Read the model definition and answer for the solid it produces. Units are mm, in the model's axes. Face numbers are marked on the shaded views. A direction names the side the tool comes from. Coordinates: 2 decimals unless noted, no trailing zeros. Write each loop counter-clockwise with the first axis right and the second up, starting at its lowest first coordinate (ties: lowest second). Pieces come first, ordered by that corner, then holes. Notation, with made-up numbers: (54, 1.5) -> (85, 1.5) arc R25 cw to (85, 30.5) -> close; hole circle Ø11 at (89, 28.5). An arc over 180 degrees is marked (long way). Answer as a JSON object with one key per item and string values. Group by question number.
(1) Which of the six approach directions +Z, -Z, +X, -X, +Y, -Y give full straight-line access (tool end or side, diameter ignored) to the marked faces 1, 2, 3, 4 and 5?
(2) Flat-ended cylindrical pins translate along their axes: P1, Ø16, axis at y = -88.5, z = 18.5, coming from the +X side; P2, Ø3, axis at y = 41, z = 138.5, coming from the -X side; P3, Ø16, axis at x = 71, z = 15, coming from the -Y side. Find the tip coordinate at first contact, or state that the pin passes through.
(3) For a pull along X with two mould halves and no side action, classify the marked faces 6, 7, 8 and 9 as +X half, -X half, draft (parallel to the pull), parting line (faces both ways), or undercut.
(4) Find section D-D (x = -63.5). Give the vertices of the cut face in (y, z), then the cut area to 3 significant figures.
(5) Find section B-B (x = 75). Give the vertices of the cut face in (y, z).
(6) Find section C-C (z = 61). Give the vertices of the cut face in (x, y).
(7) Straight lines are drawn through the part: L1, parallel to Y at x = 75, z = 11; L2, parallel to X at y = -82, z = 32; L3, parallel to Z at x = 76, y = 56. For each, find the intervals that lie inside material, in ascending order.
(8) Find section A-A (y = -82.5). Give the vertices of the cut face in (x, z), then the cut area to 3 significant figures.
from build123d import *

# Parameters (mm, degrees)
F0_W            = 210
F0_H            = 225
F1_DEPTH        = 25
F3_DEPTH        = 95
F4_R            = 37.5
F5_DEPTH        = 10
F5_DEPTH_BACK   = 127
F6_R            = 40
F7_DEPTH        = 10
F7_DEPTH_BACK   = 127
F8_W            = 60
F8_H            = 60
F9_DEPTH        = 10
F10_R           = 10
F12_DEPTH       = 20
F14_D           = 15
F14_CBORE_D     = 30
F14_CBORE_DEPTH = 10
F15_R           = 10
F16_R           = 19.5
F17_DEPTH       = 235.001
F18_R           = 19.5
F19_DEPTH       = 220.001
F20_SIZE        = 2
F21_R           = 10


with BuildPart() as f1:
    # F0 (on Top) → F1 (new body)
    with BuildSketch(Plane.XY):
        Rectangle(F0_W, F0_H)
    extrude(amount=F1_DEPTH)

    # F2 (on face) → F3 (join)
    with BuildSketch(Plane.XY.offset(25)):
        with BuildLine():
            Line((-71, -32.5), (-71, -112.5))
            Line((-71, -112.5), (-56, -112.5))
            Line((-56, -112.5), (-56, -46.481817))
            ThreePointArc((-56, -46.481817), (7.488853, -14.988853), (38.981817, 48.5))
            Line((38.981817, 48.5), (105, 48.5))
            Line((105, 48.5), (105, 63.5))
            Line((105, 63.5), (25, 63.5))
            ThreePointArc((25, 63.5), (-3.117749, -4.382251), (-71, -32.5))
        make_face()
    extrude(amount=F3_DEPTH)

    # F4 (on face) → F5 (join, two sides)
    with BuildSketch(Plane.XZ.offset(112.5)) as f5_sk:
        with Locations((-63.5, 120)):
            Circle(F4_R)
    extrude(amount=F5_DEPTH)
    extrude(f5_sk.sketch, amount=-F5_DEPTH_BACK)

    # F6 (on face) → F7 (join, two sides)
    with BuildSketch(Plane.YZ.offset(105)) as f7_sk:
        with Locations((56, 120)):
            Circle(F6_R)
    extrude(amount=F7_DEPTH)
    extrude(f7_sk.sketch, amount=-F7_DEPTH_BACK)

    # F8 (on face) → F9 (join)
    with BuildSketch(Plane.XY.offset(25)):
        with Locations((75, -82.5)):
            Rectangle(F8_W, F8_H)
    extrude(amount=F9_DEPTH)

    # F10
    f10_edges = [f1.edges().sort_by_distance(p)[0] for p in [
        (45, -52.5, 30),
    ]]
    fillet(f10_edges, radius=F10_R)

    # F11 (on face) → F12 (cut)
    with BuildSketch(Plane.XY.offset(25)):
        with BuildLine():
            ThreePointArc((46.575508, 39.5), (13.852814, -21.352814), (-47, -54.075508))
            Line((-47, -54.075508), (-47, -103.5))
            Line((-47, -103.5), (36, -103.5))
            Line((36, -103.5), (36, -62.5))
            ThreePointArc((36, -62.5), (41.564971, -49.064971), (55, -43.5))
            Line((55, -43.5), (96, -43.5))
            Line((96, -43.5), (96, 39.5))
            Line((96, 39.5), (46.575508, 39.5))
        make_face()
    extrude(amount=-F12_DEPTH, mode=Mode.SUBTRACT)

    # F14 (through all)
    with Locations(Plane.XY.offset(35)):
        with Locations((75, -82.5)):
            CounterBoreHole(F14_D / 2, F14_CBORE_D / 2, F14_CBORE_DEPTH)

    # F15
    f15_edges = [f1.edges().sort_by_distance(p)[0] for p in [
        (-47, -54.075508, 15),
        (46.575508, 39.5, 15),
        (96, 39.5, 15),
        (36, -103.5, 15),
        (96, -43.5, 15),
    ]]
    fillet(f15_edges, radius=F15_R)

    # F16 (on face) → F17 (cut, through all)
    with BuildSketch(Plane.XZ.offset(122.5)):
        with Locations((-63.5, 120)):
            Circle(F16_R)
    extrude(amount=-F17_DEPTH, mode=Mode.SUBTRACT)

    # F18 (on face) → F19 (cut, through all)
    with BuildSketch(Plane.YZ.offset(115)):
        with Locations((56, 120)):
            Circle(F18_R)
    extrude(amount=-F19_DEPTH, mode=Mode.SUBTRACT)

    # F20
    f20_edges = [f1.edges().sort_by_distance(p)[0] for p in [
        (-83, -122.5, 120),
        (115, 36.5, 120),
        (-83, 14.5, 120),
        (-22, 36.5, 120),
    ]]
    chamfer(f20_edges, length=F20_SIZE)

    # F21
    f21_edges = [f1.edges().sort_by_distance(p)[0] for p in [
        (105, -112.5, 17.5),
        (-105, -112.5, 12.5),
        (105, 112.5, 12.5),
        (-105, 112.5, 12.5),
    ]]
    fillet(f21_edges, radius=F21_R)


solid = f1.part
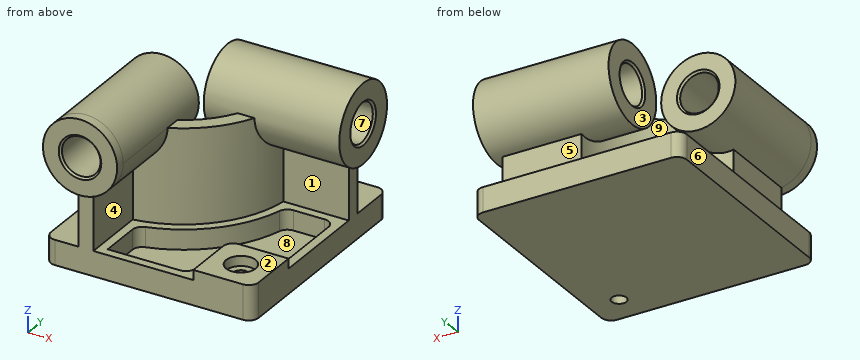
Results below:
{
 "1": {"face 1": "+X", "face 2": "+Z, +X, -Y", "face 3": "+Z, -X, +Y", "face 4": "-Y", "face 5": "+X, -X, +Y"},
 "2": {"P1": "stops at x = 105", "P2": "stops at x = -22", "P3": "stops at y = -112.5"},
 "3": {"face 6": "-X half", "face 7": "draft", "face 8": "undercut", "face 9": "undercut"},
 "4": {"outline": "(-122.5, 82.5) -> (-112.5, 82.5) -> (-112.5, 0) -> (112.5, 0) -> (112.5, 25) -> (-32.21, 25) -> (-32.21, 82.5) -> (14.5, 82.5) -> (14.5, 98.5) -> (12.5, 100.5) -> (-120.5, 100.5) -> (-122.5, 98.5) -> close; (-122.5, 141.5) -> (-120.5, 139.5) -> (12.5, 139.5) -> (14.5, 141.5) -> (14.5, 157.5) -> (-122.5, 157.5) -> close", "area": "15,200 mm2"},
 "5": {"outline": "(-112.5, 0) -> (-90, 0) -> (-90, 25) -> (-97.5, 25) -> (-97.5, 35) -> (-112.5, 35) -> close; (-75, 0) -> (112.5, 0) -> (112.5, 25) -> (63.5, 25) -> (63.5, 80.71) arc R40 ccw (long way) to (48.5, 80.71) -> (48.5, 25) -> (39.5, 25) -> (39.5, 5) -> (-43.5, 5) -> (-43.5, 25) -> (-52.5, 25) -> (-52.5, 35) -> (-67.5, 35) -> (-67.5, 25) -> (-75, 25) -> close; hole circle Ø39 at (56, 120)"},
 "6": {"outline": "(-71, -112.5) -> (-56, -112.5) -> (-56, -46.48) arc R111 ccw to (38.98, 48.5) -> (105, 48.5) -> (105, 63.5) -> (25, 63.5) arc R96 cw to (-71, -32.5) -> close"},
 "7": {"L1": "y = -112.5 to -90, -75 to -43.5, 39.5 to 112.5", "L2": "x = -71 to -56, 45 to 60.01, 89.99 to 105", "L3": "z = 0 to 100.5, 139.5 to 160"},
 "8": {"outline": "(-105, 0) -> (67.5, 0) -> (67.5, 25) -> (60, 25) -> (60, 35) -> (45, 35) -> (45, 25) -> (36, 25) -> (36, 5) -> (-47, 5) -> (-47, 25) -> (-56, 25) -> (-56, 83.26) arc R37.5 ccw (long way) to (-71, 83.26) -> (-71, 25) -> (-105, 25) -> close; (82.5, 0) -> (105, 0) -> (105, 35) -> (90, 35) -> (90, 25) -> (82.5, 25) -> close; hole circle Ø39 at (-63.5, 120)", "area": "7,600 mm2"}
}
